Input: part model. Units: mm. Frame: model coordinates. Face numbers are marked on the shaded views. A direction names the side the tool comes from. Give positions to 0.01 mm unless a question says otherwise; leave off trailing zeros. Loops run counter-clockwise (first coordinate to the right, second up) from the corner with the lowest first, then second, coordinate; pieces in that order, holes last. Notation, with made-up numbers: (7.25, 48) -> (57.25, 48) arc R19 ccw to (57.25, 75) -> close; hole circle Ø7 at (-14.75, 42). An arc over 180 degrees is marked (long way). Answer as a JSON object with one key per item and string values.
```python
from build123d import *

# Parameters (mm, degrees)
SKETCH017_R     = 1.65
SKETCH017_W     = 30
SKETCH017_H     = 38
PAD012_DEPTH    = 22
POCKET057_DEPTH = 41.001
POCKET058_DEPTH = 40.001


with BuildPart() as part:
    # Sketch017 → Pad012 (new body)
    with BuildSketch(Plane.XY):
        with BuildLine():
            Line((-16.5, 18.5), (16.5, 18.5))
            Line((16.5, 18.5), (16.5, 32))
            ThreePointArc((20, 35.5), (17.525126, 34.474874), (16.5, 32))
            ThreePointArc((20, 35.5), (23.5, 39), (20, 42.5))
            ThreePointArc((16.5, 46), (17.525126, 43.525126), (20, 42.5))
            Line((16.5, 59.5), (16.5, 46))
            Line((-16.5, 59.5), (16.5, 59.5))
            Line((-16.5, 59.5), (-16.5, 46))
            ThreePointArc((-20, 42.5), (-17.525126, 43.525126), (-16.5, 46))
            ThreePointArc((-20, 42.5), (-23.5, 39), (-20, 35.5))
            ThreePointArc((-16.5, 32), (-17.525126, 34.474874), (-20, 35.5))
            Line((-16.5, 18.5), (-16.5, 32))
        make_face()
        with Locations((-20, 39)):
            Circle(SKETCH017_R, mode=Mode.SUBTRACT)
        with Locations((20, 39)):
            Circle(SKETCH017_R, mode=Mode.SUBTRACT)
        with Locations((0, 39)):
            Rectangle(SKETCH017_W, SKETCH017_H, mode=Mode.SUBTRACT)
    extrude(amount=PAD012_DEPTH)

    # Sketch111 (on Face7 of Pad012) → Pocket057 (cut, through all)
    with BuildSketch(Plane(origin=(0, 59.5, 0), x_dir=(-1, 0, 0), z_dir=(0, 1, 0))):
        Polygon((-15, 2.710372), (-8.455557, 11), (-15, 19.289628), align=None)
        Polygon((-14.044443, 1.5), (-7.5, 9.789628), (-0.955557, 1.5), align=None)
        Polygon((-14.044443, 20.5), (-0.955557, 20.5), (-7.5, 12.210372), align=None)
        Polygon((-6.544443, 11), (0, 19.289628), (6.544443, 11), (0, 2.710372), align=None)
        Polygon((0.955557, 1.5), (7.5, 9.789628), (14.044443, 1.5), align=None)
        Polygon((8.455557, 11), (15, 2.710372), (15, 19.289628), align=None)
        Polygon((7.5, 12.210372), (0.955557, 20.5), (14.044443, 20.5), align=None)
    extrude(amount=-POCKET057_DEPTH, mode=Mode.SUBTRACT)

    # Sketch112 (on Face2 of Pocket057) → Pocket058 (cut, through all)
    with BuildSketch(Plane(origin=(-16.5, 0, 0), x_dir=(0, -1, 0), z_dir=(-1, 0, 0))):
        Polygon((-56.791693, 1.5), (-46, 10.043423), (-46, 1.5), align=None)
        Polygon((-58, 2.456577), (-58, 19.543423), (-47.208307, 11), align=None)
        Polygon((-32, 1.5), (-32, 10.043423), (-21.208307, 1.5), align=None)
        Polygon((-32, 20.5), (-32, 11.956577), (-21.208307, 20.5), align=None)
        Polygon((-30.791693, 11), (-20, 19.543423), (-20, 2.456577), align=None)
        Polygon((-46, 11.956577), (-46, 20.5), (-56.791693, 20.5), align=None)
    extrude(amount=-POCKET058_DEPTH, mode=Mode.SUBTRACT)


with BuildPart() as part_1:
    # Body011 placement: moved
    add(part.part.moved(Location((0, 0, 59.7))))


solid = part_1.part
```
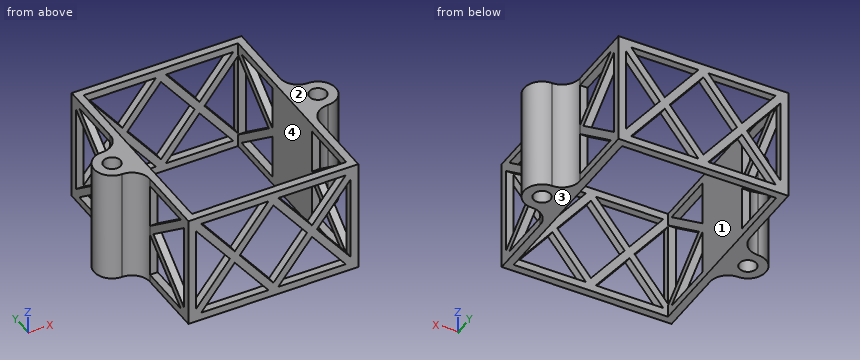
Q1. Draft query along X for the marked faces 3 and 4. Return one class per face: +X half, -X half, draft (parallel to the pull), parting line (faces both ways), or undercut.
Evaluation:
{"face 3": "draft", "face 4": "undercut"}
Q2. Section B-B, the plane x = 10.5. Give the number of separate pieces and of enclosed holes in the cut face, then the cut area to 3 significant figures.
Evaluation:
{"separate pieces": "8", "enclosed holes": "0", "area": "23.5 mm2"}
Q3. Pin query (flat end, axial travel): pin 1 (1 mm diameter, centred on x = -14.5, z = 78, fed in from +Y); pin 2 (1.6 mm diameter, centred on y = 19, z = 73, fed in from -X); pin 3 (7 mm diameter, centred on y = 53.5, z = 73.5, fed in from +X); pin 4 (1.5 mm diameter, centred on y = 42.5, z = 72, fed in from -X). Return the tip coordinate at first contact, or that it passes through.
Evaluation:
{"pin 1": "stops at y = 59.5", "pin 2": "stops at x = -16.5", "pin 3": "stops at x = 16.5", "pin 4": "stops at x = -22.17"}
Q4. Ray query, line 1 along Y through (x, z) = (-8, 69.25); line 2 along Y through (x, z) = (-20, 71.5); line 3 along X through (y, z) = (29, 80.5). Return the intervals inside material, ascending.
Evaluation:
{"line 1": "y = 18.5 to 20, 58 to 59.5", "line 2": "y = 35.5 to 37.35, 40.65 to 42.5", "line 3": "x = -16.5 to -15, 15 to 16.5"}
Q5. Access query for the marked faces 1 and 2. Directions: +Z, -Z, +X, -X, +Y, -Y. A direction counts if a zero-diameter tool reaches every point of the face in a straight line with its end or side. Return the directions, or none.
Evaluation:
{"face 1": "+Z, -Z", "face 2": "+Z, +X, -X, +Y, -Y"}
Q6. Section A-A, the plane y = 44.5. Return the cut outline in (x, z), then the cut area to 3 significant figures.
Evaluation:
{"outline": "(-16.84, 59.7) -> (-15, 59.7) -> (-15, 81.7) -> (-16.84, 81.7) -> close; (15, 59.7) -> (16.84, 59.7) -> (16.84, 81.7) -> (15, 81.7) -> close", "area": "80.9 mm2"}
